Verification items for the finished model (mm, model axes). A direction names the side the tool comes from. Coordinates: 2 decimals unless noted, no trailing zeros. Order: outer loops, then holes, each group sorted by start corner. A loop starts at its lowest first (then second) coordinate and runs counter-clockwise, first axis right, second up. Notation, with made-up numbers: (-24, -37) -> (24, -37) arc R21 ccw to (24, -22) -> close; hole circle Ø1 at (6, 82.5). An arc over 180 degrees is marked (long way). Write item = value, one per line. Start each with the question number.
1. Thickness scan on line 1 along Z through (x, y) = (-4.5, -27); line 2 along Z through (x, y) = (-3, -46.5); line 3 along X through (y, z) = (30.5, -9). Record the ranges inside material, lowest first. Write a range as from..to.
2. Release check for a two-part mould opening along Z. For faces 4 (the flat face through (0, 62, -6)), 5 (the flat face through (5, -11, -13)), 6 (the flat face through (0, -77, -26)) record: +Z half, -Z half, draft (parallel to the pull), parting line (faces both ways), or undercut.
3. Set-up check for faces 1 (the cylindrical face through (4.4, -29.51, -14.79)), 2 (the cylindrical face through (-4.4, -29.51, -14.79)), 3 (the flat face through (0.04, -35.5, -15.86)): record each of +Z, -Z, +X, -X, +Y, -Y from which the full face is reachable in a straight line by a thin tool's end or side.
4. Cross-section at B-B on x = -0.5. Record the cut outline in (y, z), plus the area to 3 significant figures.
5. Cross-section at A-A on y = 58.5. Record the cut outline in (x, z), plus the area to 3 significant figures.
6. Go/stop test with flat-tipped pins: P1, Ø1.8, axis at x = 1.5, y = -54.5, coming from the -Z side; P2, Ø1.5, axis at x = 3, y = 10, coming from the -Z side; P3, Ø2, axis at x = -4, y = -42.5, coming from the -Z side. Record where each tip stops, or that it passes through.
from build123d import *

# Parameters (mm, degrees)
SKETCH1_W           = 12
SKETCH1_H           = 164
BOSS_EXTRUDE1_DEPTH = 5
FILLET1_R           = 2


with BuildPart() as part:
    # Sketch1 → Boss-Extrude1 (new, symmetric)
    with BuildSketch(Plane(origin=(0, 0, 0), x_dir=(0, 0, -1), z_dir=(1, 0, 0))):
        Polygon((38, -72), (6, 43.2), (6, 0), (26, -72), (26, -82), (38, -82), align=None)
        Rectangle(SKETCH1_W, SKETCH1_H)
    extrude(amount=BOSS_EXTRUDE1_DEPTH, both=True)

    # Fillet1
    fillet1_edges = [part.edges().sort_by_distance(p)[0] for p in [
        (5, -77, -26),
        (-5, -41, -6),
        (-5, -82, 0),
        (-5, 0, 6),
        (-5, 82, 0),
        (-5, 62.6, -6),
        (-5, -14.4, -22),
        (-5, -77, -38),
        (5, -82, -32),
        (-5, -82, -32),
        (-5, -77, -26),
        (-5, -36, -16),
        (5, -77, -38),
        (5, -14.4, -22),
        (5, 62.6, -6),
        (5, 82, 0),
        (5, 0, 6),
        (5, -82, 0),
        (5, -36, -16),
        (5, -41, -6),
    ]]
    fillet(fillet1_edges, radius=FILLET1_R)


solid = part.part
Worked out:
q1.line_1 = -24.8..-14.2, -5.32..5.32
q1.line_2 = -30.92..-18.92, -6..6
q1.line_3 = -4.33..4.33
q2.face_4 = -Z half
q2.face_5 = draft
q2.face_6 = undercut
q3.face_1 = +X, -Y
q3.face_2 = -X, -Y
q3.face_3 = +X, -X, -Y
q4.outline = (-82, -38) -> (-72, -38) -> (43.2, -6) -> (82, -6) -> (82, 6) -> (-82, 6) -> (-82, -6) -> (0, -6) -> (-72, -26) -> (-82, -26) -> close
q4.area = 3,210 mm²
q5.outline = (-5, -4) arc R2 ccw to (-3, -6) -> (3, -6) arc R2 ccw to (5, -4) -> (5, 4) arc R2 ccw to (3, 6) -> (-3, 6) arc R2 ccw to (-5, 4) -> close
q5.area = 117 mm²
q6.P1 = -33.39
q6.P2 = -15.43
q6.P3 = -29.99
